Can you work these out from the model? Positions are in its coordinate system, mm. A direction names the side the tool comes from. Give positions to 0.01 mm unless a question says otherwise; leave off trailing zeros. Loops run counter-clockwise (first coordinate to the right, second up) from the corner with the lowest first, then second, coordinate; pieces in that order, holes last. Notation, with made-up numbers: (-12.5, -14) -> (13.5, -14) arc R18 cw to (13.5, 13) -> close; hole circle Ø9 at (32, -2). An arc over 180 degrees is marked (long way). Return JSON: item names as keys, results as strings. Group by question number.
Q1. I need wall thicknesses on line 1 along Y through (x, z) = (17, 71.5); line 2 along Z through (x, y) = (26.5, -35.5). Which ranges of each line are inside material? Lowest first, please. Write a range as [from, to].
Q2. Will this pin go through, and if not, where does the flat tip stop? pin 1 (8 mm diameter, centred on x = -21, y = 14, fed in from -Z).
Q3. Suppose I cut it at B-B, the plane y = -9. Please give me the cut outline in (x, z), and give its area (3 significant figures).
Q4. Which directions (+Z, -Z, +X, -X, +Y, -Y) give clear straight access to the entire face, cutting with the end or side of a thin tool? Please do faces 4 (the flat face through (-38, -1, 38)), 5 (the flat face through (-1, 1, 80)).
Q5. Thinking about a two-plate mould opening in Y: for faces 1 (the flat face through (-40, 1, 39)), 2 (the flat face through (33, -34, 39)), 3 (the flat face through (-5, -38, 38)), which applies, pulls with the +Y half, pulls with the -Y half, needs draft (parallel to the pull), parting line crosses it, or undercut?
Q6. Suppose I cut it at A-A, the plane z = 12.5. Please give me the cut outline in (x, y), and give its area (3 significant figures).
```python
from build123d import *

# Parameters (mm, degrees)
BOSS_EXTRU_1_DEPTH      = 80
ENL_V_MAT_EXTRU_1_DEPTH = 78


with BuildPart() as part:
    # Esquisse1 → Boss.-Extru.1 (new body)
    with BuildSketch(Plane.XY):
        Polygon((27, -40), (40, -27), (40, 40), (-40, 40), (-40, -40), align=None)
    extrude(amount=BOSS_EXTRU_1_DEPTH)

    # Esquisse2 → Enlèv. mat.-Extru.1 (cut)
    with BuildSketch(Plane(origin=(0, 0, 0), x_dir=(-1, 0, 0), z_dir=(0, 0, -1))):
        Polygon((-38, -26.171572875), (-26.171572875, -38), (38, -38), (38, 38), (-38, 38), align=None)
    extrude(amount=-ENL_V_MAT_EXTRU_1_DEPTH, mode=Mode.SUBTRACT)


solid = part.part
```
Ans:
{
 "1": {"line 1": "y = [-40, -38], [38, 40]", "line 2": "z = [78, 80]"},
 "2": {"pin 1": "stops at z = 78"},
 "3": {"outline": "(-40, 0) -> (-38, 0) -> (-38, 78) -> (38, 78) -> (38, 0) -> (40, 0) -> (40, 80) -> (-40, 80) -> close", "area": "472 mm^2"},
 "4": {"face 4": "-Z", "face 5": "+Z, +X, -X, +Y, -Y"},
 "5": {"face 1": "needs draft", "face 2": "pulls with the -Y half", "face 3": "undercut"},
 "6": {"outline": "(-40, -40) -> (27, -40) -> (40, -27) -> (40, 40) -> (-40, 40) -> close; hole (-38, -38) -> (26.17, -38) -> (38, -26.17) -> (38, 38) -> (-38, 38) -> close", "area": "609 mm^2"}
}
